Read the model definition and answer for the solid it produces. Units are mm, in the model's axes. A direction names the side the tool comes from. Round coordinates to 2 decimals unless told otherwise and drop trailing zeros. Write each loop counter-clockwise with the first axis right and the second up, starting at its lowest first coordinate (ties: lowest second). Pieces come first, ordered by that corner, then holes. Notation, with made-up numbers: (75.25, 15) -> (127.25, 15) arc R17 ccw to (127.25, 43) -> close; hole circle Ø10 at (84.25, -20.5). An arc over 180 degrees is marked (long way). Return JSON: item names as keys, results as strings. Group by question number.
(1) The mould has two halves that part along X. Classify faces 3 (the cylindrical face through (0.3, -1.7, 12.6)), 4 (the conical face through (-4.724, 29.706, 57.114)), 5 (the flat face through (-18.256, 1, 15)): released by +X, released by -X, zero draft, split by the parting line, or undercut.
(2) Given pin 1 (10 mm diameter, centred on x = -9.5, y = -34, fed in from -Z); pin 2 (23 mm diameter, centred on y = 0, z = 0, fed in from +X); pin 3 (5 mm diameter, centred on x = -1.5, y = -49, fed in from -Z); pin 4 (1.5 mm diameter, centred on x = 13, y = 33.5, fed in from +Z), each flat-ended and moving along its own axis, determine where each tip first touches the part or whether it passes through.
(3) Straight lines are drawn through the part: line 1 (Z direction, x = -1, y = 0); line 2 (X direction, y = -6, z = 62.5); line 3 (X direction, y = 45, z = -41.5). For each, find the intervals that lie inside material, in ascending order.
(4) A cutting plane is placed at C-C on x = 0. Give the vertices of the cut face in (y, z) (3 decimals).
(5) For faces 1 (the cylindrical face through (11.984, -15.485, 69.733)), 2 (the conical face through (4.75, -13.98, 62.95)), determine the directions among +Z, -Z, +X, -X, +Y, -Y from which every point of the face is accessible in a straight line to the end or side of a thin tool.
```python
from build123d import *

# Parameters (mm, degrees)
SKETCH2_R          = 12.7127
CUT_EXTRUDE1_DEPTH = 37.5125


with BuildPart() as part:
    # Sketch1 → Revolve1 (revolve)
    with BuildSketch(Plane.XY):
        with BuildLine():
            Line((18.25625, 0), (-18.25625, 0))
            Line((-18.25625, 0), (-18.25625, 70.6374))
            Line((-18.25625, 70.6374), (-17.4625, 71.43115))
            Line((-17.4625, 71.43115), (-6.35, 71.43115))
            Line((-6.35, 71.43115), (-4.640755559, 64.017549491))
            ThreePointArc((-4.640755559, 64.017549491), (0, 60.325), (4.640755559, 64.017549491))
            Line((4.640755559, 64.017549491), (6.35, 71.43115))
            Line((6.35, 71.43115), (17.4625, 71.43115))
            Line((17.4625, 71.43115), (18.25625, 70.6374))
            Line((18.25625, 70.6374), (18.25625, 0))
        make_face()
    revolve(axis=Axis((18.25625, 0, 0), (-1, 0, 0)))

    # Sketch2 → Cut-Extrude1 (cut, through all)
    with BuildSketch(Plane(origin=(18.25625, 0, 0), x_dir=(0, 0, -1), z_dir=(1, 0, 0))):
        with Locations(Location((0, 0, 0), (0, 0, 90))):  # turned: the seam where the file's is
            Circle(SKETCH2_R)
    extrude(amount=-CUT_EXTRUDE1_DEPTH, mode=Mode.SUBTRACT)


solid = part.part
```
Checks:
{
 "1": {"face 3": "zero draft", "face 4": "undercut", "face 5": "released by -X"},
 "2": {"pin 1": "stops at z = -65.28", "pin 2": "passes through", "pin 3": "stops at z = -39.63", "pin 4": "stops at z = 63.48"},
 "3": {"line 1": "z = -60.43 to -12.71, 12.71 to 60.43", "line 2": "x = -18.26 to -4.17, 4.17 to 18.26", "line 3": "x = -18.26 to -2.77, 2.77 to 18.26"},
 "4": {"outline": "circle Ø120.65 at (0, 0); hole circle Ø25.425 at (0, 0)"},
 "5": {"face 1": "+X, -X", "face 2": "none"}
}
